from build123d import *

# Parameters (mm, degrees)
SKETCH4_W                = 25
SKETCH4_H                = 7
BOSS_EXTRUDE3_DEPTH      = 3
BOSS_EXTRUDE3_DEPTH_BACK = 3
FILLET2_R                = 8
CUT_EXTRUDE1_REACH       = 73.009


with BuildPart() as part:
    # Sketch4 → Revolve2 (revolve)
    with BuildSketch(Plane(origin=(0, 0, 0), x_dir=(1, 0, 0), z_dir=(0, 1, 0)), mode=Mode.PRIVATE) as revolve2_sk:
        with Locations((37.5, 0)):
            Rectangle(SKETCH4_W, SKETCH4_H)
    revolve(revolve2_sk.sketch.rotate(Axis((0, 0, -11.674254949), (0, 0, 1)), 180), axis=Axis((0, 0, -11.674254949), (0, 0, 1)))

    # Sketch5 → Boss-Extrude3 (add, two sides: drawn at the far end of the back side and taken through both)
    with BuildSketch(Plane.XY.offset(-BOSS_EXTRUDE3_DEPTH_BACK)):
        with BuildLine():
            Line((-3, 24.819347292), (-3, 3))
            Line((-3, 3), (-24.819347292, 3))
            ThreePointArc((-24.819347292, 3), (-25, 0), (-24.819347292, -3))
            Line((-24.819347292, -3), (-3, -3))
            Line((-3, -3), (-3, -24.819347292))
            ThreePointArc((-3, -24.819347292), (0, -25), (3, -24.819347292))
            Line((3, -24.819347292), (3, -3))
            Line((3, -3), (24.819347292, -3))
            ThreePointArc((24.819347292, -3), (25, 0), (24.819347292, 3))
            Line((24.819347292, 3), (3, 3))
            Line((3, 3), (3, 24.819347292))
            ThreePointArc((3, 24.819347292), (0, 25), (-3, 24.819347292))
        make_face()
    extrude(amount=BOSS_EXTRUDE3_DEPTH + BOSS_EXTRUDE3_DEPTH_BACK)

    # Fillet2
    fillet2_edges = [part.edges().sort_by_distance(p)[0] for p in [
        (-3, 24.819347292, 0),
        (3, 24.819347292, 0),
        (3, 3, 0),
        (24.819347292, 3, 0),
        (24.819347292, -3, 0),
        (3, -3, 0),
        (3, -24.819347292, 0),
        (-3, -24.819347292, 0),
        (-3, -3, 0),
        (-24.819347292, -3, 0),
        (-24.819347292, 3, 0),
        (-3, 3, 0),
    ]]
    fillet(fillet2_edges, radius=FILLET2_R)

    # Sketch6 → Cut-Extrude1 (cut, up to next)
    with BuildSketch(Plane.XY.offset(3), mode=Mode.PRIVATE) as cut_extrude1_sk1:
        with BuildLine():
            Line((1, 1.118033989), (1, -1.118033989))
            ThreePointArc((1, -1.118033989), (-1.5, 0), (1, 1.118033989))
        make_face()
    cut_extrude1_tool1 = extrude(cut_extrude1_sk1.sketch, amount=-CUT_EXTRUDE1_REACH, mode=Mode.PRIVATE) & part.part
    add(cut_extrude1_tool1.solids().sort_by_distance((-0.148024, 0, 3))[0], mode=Mode.SUBTRACT)


solid = part.part
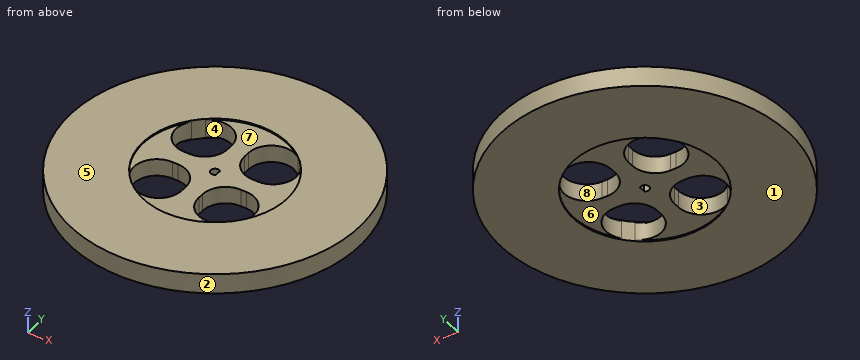
Input: part model. Units: mm. Frame: model coordinates. Face numbers are marked on the shaded views. A direction names the side the tool comes from. Coordinates: 2 decimals unless noted, no trailing zeros. Loops run counter-clockwise (first coordinate to the right, second up) from the corner with the lowest first, then second, coordinate; pieces in that order, holes last.
(1) Set-up query: the marked faces 5, 6, 7 and 8. Return all of +Z, -Z, +X, -X, +Y, -Y with unobstructed straight access to the full face (end or side cutting, diameter ignored); none if empty.
(2) Pull-direction query (X, two-part tool) for the marked faces 1, 2, 3 and 4; classes: released by +X, released by -X, zero draft, split by the parting line, or undercut.
(3) Section B-B on z = -1.5. Return the cut outline in (x, y), then the cut area to 3 significant figures.
(4) Section C-C on x = 23. Return the cut outline in (y, z).
(5) Section A-A on y = -7.5. Return the cut outline in (x, z).
(6) First-contact query: pin 1 Ø0.6 at (y, z) = (-11.5, 0.5) entering from -X; pin 2 Ø25 at (x, y) = (8.5, 2.5) entering from -Z; pin 3 Ø0.6 at (x, z) = (-12.5, 1) entering from +Y. Flat tips, straight axial feed; report the tip coordinate or a pass-through.
(7) Section D-D on y = -39.5. Return the cut outline in (x, z).
(8) Material intervals for probe 1 along X at (y, z) = (19, -0.25); probe 2 along Y at (x, z) = (0, -0.5); probe 3 along Y at (x, z) = (-7.5, -2.5), sorted ascending.
Data:
1. face 5: +Z, +X, -X, +Y, -Y
1. face 6: -Z
1. face 7: +Z
1. face 8: +Z, -Z
2. face 1: zero draft
2. face 2: split by the parting line
2. face 3: undercut
2. face 4: undercut
3. outline: circle Ø100 at (0, 0); hole (-19.06, -16.18) arc R25 ccw to (-16.18, -19.06) arc R8 ccw to (-3, -12.96) - (-3, -11) arc R8 ccw to (-11, -3) - (-12.96, -3) arc R8 ccw to start; hole (-19.06, 16.18) arc R8 ccw to (-12.96, 3) - (-11, 3) arc R8 ccw to (-3, 11) - (-3, 12.96) arc R8 ccw to (-16.18, 19.06) arc R25 ccw to start; hole (1, -1.12) - (1, 1.12) arc R1.5 ccw (long way) to start; hole (3, -12.96) arc R8 ccw to (16.18, -19.06) arc R25 ccw to (19.06, -16.18) arc R8 ccw to (12.96, -3) - (11, -3) arc R8 ccw to (3, -11) - close; hole (3, 11) arc R8 ccw to (11, 3) - (12.96, 3) arc R8 ccw to (19.06, 16.18) arc R25 ccw to (16.18, 19.06) arc R8 ccw to (3, 12.96) - close
3. area: 6,820 mm2
4. outline: (-44.4, -3.5) - (-9.8, -3.5) - (-9.8, -3) - (9.8, -3) - (9.8, -3.5) - (44.4, -3.5) - (44.4, 3.5) - (9.8, 3.5) - (9.8, 3) - (-9.8, 3) - (-9.8, 3.5) - (-44.4, 3.5) - close
5. outline: (-49.43, -3.5) - (-23.85, -3.5) - (-23.85, -3) - (-20.16, -3) - (-20.16, 3) - (-23.85, 3) - (-23.85, 3.5) - (-49.43, 3.5) - close; (-3.81, -3) - (3.81, -3) - (3.81, 3) - (-3.81, 3) - close; (20.16, -3) - (23.85, -3) - (23.85, -3.5) - (49.43, -3.5) - (49.43, 3.5) - (23.85, 3.5) - (23.85, 3) - (20.16, 3) - close
6. pin 1: stops at x = -48.73
6. pin 2: stops at z = -3
6. pin 3: stops at y = 48.49
7. outline: (-30.66, -3.5) - (30.66, -3.5) - (30.66, 3.5) - (-30.66, 3.5) - close
8. probe 1: x = -46.25 to -16.25, -5.75 to 5.75, 16.25 to 46.25
8. probe 2: y = -50 to -1.5, 1.5 to 50
8. probe 3: y = -49.43 to -20.16, -3.81 to 3.81, 20.16 to 49.43
